Work out the finished part from the listing and answer in its coordinate system (mm). A direction names the side the tool comes from. Round coordinates to 2 decimals unless told otherwise and drop trailing zeros. Loops run counter-clockwise (first coordinate to the right, second up) from the corner with the lowest first, then second, coordinate; pieces in that order, holes last. Notation, with made-up numbers: (9, 53.25) - (20, 53.25) arc R29 cw to (20, 83.25) - close; hole circle Ø3 at (-13.5, -35). An arc over 180 degrees is marked (long way). Use CSV: the item, a comma, the result in double quotes. Start each with the question number.
from build123d import *

# Parameters (mm, degrees)
SKETCH1_W               = 50
SKETCH1_H               = 15.4
SKETCH1_W_2             = 36
SKETCH1_H_2             = 1.5
BOSS_EXTRUDE1_DEPTH     = 1.5
SKETCH2_W               = 9.6
SKETCH2_H               = 2
SKETCH2_W_2             = 4.5
BOSS_EXTRUDE2_DEPTH     = 2.5
CHAMFER3_SIZE           = 1.5
CHAMFER4_SIZE           = 1.5
FILLET3_R               = 1.4
SKETCH5_W               = 9.6
SKETCH5_H               = 1.5
BOSS_EXTRUDE4_DEPTH     = 2
FILLET4_R               = 1.4
SKETCH6_W               = 4.5
SKETCH6_H               = 1.5
BOSS_EXTRUDE5_DEPTH     = 1.5
FILLET5_R               = 1.4
CUT_EXTRUDE5_DEPTH      = 88.490987959
CUT_EXTRUDE5_DEPTH_BACK = 88.490987959


with BuildPart() as part:
    # Sketch1 → Boss-Extrude1 (new body)
    with BuildSketch(Plane(origin=(0, 0, 0), x_dir=(1, 0, 0), z_dir=(0, 1, 0))):
        with Locations((-61.287356322, 5.044827586)):
            Rectangle(SKETCH1_W, SKETCH1_H)
        with Locations((-61.287356322, 0.094827586)):
            Rectangle(SKETCH1_W_2, SKETCH1_H_2, mode=Mode.SUBTRACT)
    extrude(amount=BOSS_EXTRUDE1_DEPTH)

    # Sketch2 → Boss-Extrude2 (add)
    with BuildSketch(Plane(origin=(0, 1.5, 0), x_dir=(1, 0, 0), z_dir=(0, 1, 0))):
        with Locations((-61.487356322, -1.655172414)):
            Rectangle(SKETCH2_W, SKETCH2_H)
        with Locations((-75.037356322, 11.744827586)):
            Rectangle(SKETCH2_W_2, SKETCH2_H)
        with Locations((-47.537356322, 11.744827586)):
            Rectangle(SKETCH2_W_2, SKETCH2_H)
    extrude(amount=BOSS_EXTRUDE2_DEPTH)

    # Chamfer3
    chamfer3_edges = [part.edges().sort_by_distance(p)[0] for p in [
        (-75.037356322, 4, -10.744827586),
    ]]
    chamfer(chamfer3_edges, length=CHAMFER3_SIZE)

    # Chamfer4
    chamfer4_edges = [part.edges().sort_by_distance(p)[0] for p in [
        (-61.487356322, 4, 0.655172414),
        (-47.537356322, 4, -10.744827586),
    ]]
    chamfer(chamfer4_edges, length=CHAMFER4_SIZE)

    # Fillet3
    fillet3_edges = [part.edges().sort_by_distance(p)[0] for p in [
        (-75.037356322, 2.5, -10.744827586),
        (-47.537356322, 2.5, -10.744827586),
    ]]
    fillet(fillet3_edges, radius=FILLET3_R)

    # Sketch5 → Boss-Extrude4 (add)
    with BuildSketch(Plane.XY.offset(2.655172414)):
        with Locations((-61.487356322, 3.25)):
            Rectangle(SKETCH5_W, SKETCH5_H)
    extrude(amount=BOSS_EXTRUDE4_DEPTH)

    # Fillet4
    fillet4_edges = [part.edges().sort_by_distance(p)[0] for p in [
        (-61.487356322, 2.5, 0.655172414),
    ]]
    fillet(fillet4_edges, radius=FILLET4_R)

    # Sketch6 → Boss-Extrude5 (add)
    with BuildSketch(Plane(origin=(0, 0, -12.744827586), x_dir=(-1, 0, 0), z_dir=(0, 0, -1))):
        with Locations((47.537356322, 3.25)):
            Rectangle(SKETCH6_W, SKETCH6_H)
        with Locations((75.037356322, 3.25)):
            Rectangle(SKETCH6_W, SKETCH6_H)
    extrude(amount=BOSS_EXTRUDE5_DEPTH)

    # Fillet5
    fillet5_edges = [part.edges().sort_by_distance(p)[0] for p in [
        (-47.537356322, 4, -14.244827586),
        (-75.037356322, 4, -14.244827586),
    ]]
    fillet(fillet5_edges, radius=FILLET5_R)

    # Sketch7 → Cut-Extrude5 (cut, two sides: drawn at the far end of the back side and taken through both)
    with BuildSketch(Plane(origin=(0, 1.5, 0), x_dir=(1, 0, 0), z_dir=(0, 1, 0)).offset(-CUT_EXTRUDE5_DEPTH_BACK)):
        with BuildLine():
            Line((-79.287356322, 0.844827586), (-43.287356322, 0.844827586))
            ThreePointArc((-43.287356322, 0.844827586), (-61.287356322, 2.968136908), (-79.287356322, 0.844827586))
        make_face()
    extrude(amount=CUT_EXTRUDE5_DEPTH + CUT_EXTRUDE5_DEPTH_BACK, mode=Mode.SUBTRACT)


solid = part.part
Item 1: A cutting plane is placed at C-C (y = 3.5). Determine the outline of the cut face in (x, z), plus the area to 3 significant figures.
Item 2: Find the intervals of material crossed by probe 1 along Y at (x, z) = (-47.5, -5.5); probe 2 along Z at (x, y) = (-76.5, 1.2); probe 3 along X at (y, z) = (1.8, 2.5), in increasing order. Write a range as [from, to].
Item 3: A cutting plane is placed at A-A (z = -1.5). Determine the outline of the cut face in (x, y), plus the area to 3 significant figures.
Item 4: A cutting plane is placed at D-D (z = -6.5). Determine the outline of the cut face in (x, y).
Item 5: Which of the six approach directions +Z, -Z, +X, -X, +Y, -Y give full straight-line access (tool end or side, diameter ignored) to faces 1 (the flat face through (-45.287, 3, -12)), 2 (the flat face through (-62, 2.5, 4)), 3 (the flat face through (-66.287, 3, 3)), 4 (the flat face through (-62, 4, 3)), 5 (the flat face through (-48, 2.5, -13))?
Item 6: The mould has two halves that part along X. Classify faces 6 (the flat face through (-36.287, 1, -5)), 7 (the cylindrical face through (-75.01, 2.45, -10.85)), 8 (the flat face through (-62, 1, 0.655)), 9 (the cylindrical face through (-61.033, 0.74, -2.968)): pulls with the +X half, pulls with the -X half, needs draft (parallel to the pull), parting line crosses it, or undercut.
Item 7: A cutting plane is placed at B-B (x = -70). Determine the outline of the cut face in (y, z), plus the area to 3 significant figures.
Item 8: Each of these flat-tipped pins is pushed along its axis until it touches: pin 1 Ø0.8 at (y, z) = (2.5, -12.5) entering from +X; pin 2 Ø0.8 at (y, z) = (3, -12.5) entering from -X; pin 3 Ø0.8 at (x, y) = (-67, 1) entering from +Z. Where does it stop, or does it pass through?
Result sheet:
1,outline,"(-77.29, -13.92) - (-72.79, -13.92) - (-72.79, -11.74) - (-77.29, -11.74) - close; (-66.29, 1.66) - (-56.69, 1.66) - (-56.69, 4.66) - (-66.29, 4.66) - close; (-49.79, -13.92) - (-45.29, -13.92) - (-45.29, -11.74) - (-49.79, -11.74) - close"
1,area,"48.4 mm^2"
2,probe 1,"[0, 1.5]"
2,probe 2,"[-12.74, -1.46], [0.66, 2.66]"
2,probe 3,"[-66.29, -56.69]"
3,outline,"(-86.29, 0) - (-76.29, 0) - (-76.29, 1.5) - (-86.29, 1.5) - close; (-46.29, 0) - (-36.29, 0) - (-36.29, 1.5) - (-46.29, 1.5) - close"
3,area,"30.0 mm^2"
4,outline,"(-86.29, 0) - (-36.29, 0) - (-36.29, 1.5) - (-86.29, 1.5) - close"
5,face 1,"+Z, -Z, +X, +Y"
5,face 2,"+Z, +X, -X, -Y"
5,face 3,"+Z, -Z, -X, +Y"
5,face 4,"+Z, -Z, +X, -X, +Y"
5,face 5,"-Z, +X, -X, -Y"
6,face 6,"pulls with the +X half"
6,face 7,"needs draft"
6,face 8,"undercut"
6,face 9,"undercut"
7,outline,"(0, -12.74) - (1.5, -12.74) - (1.5, -2.48) - (0, -2.48) - close; (0, 0.66) - (1.5, 0.66) - (1.5, 2.66) - (0, 2.66) - close"
7,area,"18.4 mm^2"
8,pin 1,"x = -45.29"
8,pin 2,"x = -77.29"
8,pin 3,"z = 2.66"
